Can you work these out from the model? Positions are in its coordinate system, mm. Face numbers are marked on the shaded views. A direction names the side the tool comes from. Give positions to 0.01 mm unless a question says otherwise; leave off trailing zeros. Order: outer loops, then holes, each group sorted by start corner. A loop starts at its lowest first (then second) coordinate and runs counter-clockwise, first axis right, second up. Notation, with made-up numbers: M -36,-8.75 L -16,-8.75 A8 ccw -16,-3.75 Z; hole C 33,75 d6. An arc over 180 degrees is marked long. One line per question, with ' | ' between items. Start each with the question number.
1) Thinking about a two-plate mould opening in Z: for the marked faces 4, 5 and 6, which applies, +Z half, -Z half, draft (parallel to the pull), parting line (faces both ways), or undercut?
2) If we section it at C-C, the plane x = 2.25: Please give me the cut outline in (y, z), plus the area to 3 significant figures.
3) If we section it at D-D, the plane y = 24: Please give me the cut outline in (x, z).
4) Please list where these lines run through material, in increasing order: line 1 along Y through (x, z) = (5.25, -4); line 2 along Y through (x, z) = (3, -7.5); line 3 along X through (y, z) = (9, -15). Write a range as [from, to].
5) I'm going to push flat-ended pins straight in: pin 1 Ø1.5 at (y, z) = (23, -5) entering from +X; pin 2 Ø1.5 at (y, z) = (7.5, -33) entering from +X; pin 3 Ø3 at (x, y) = (2, 10.5) entering from -Z; pin 4 Ø6 at (x, y) = (2, 10) entering from +Z. Where does each tip first touch, or does it pass through?
6) For the marked faces 1, 2 and 3, which set-ups out of +Z, -Z, +X, -X, +Y, -Y let a thin tool reach every point of the face, with its end or its side?
7) If we section it at B-B, the plane y = 11.25: State how many separate pieces and enclosed holes the cut face has, plus the area to 3 significant figures.
8) If we section it at A-A, the plane z = -8: Please give me the cut outline in (x, y), plus the area to 3 significant figures.
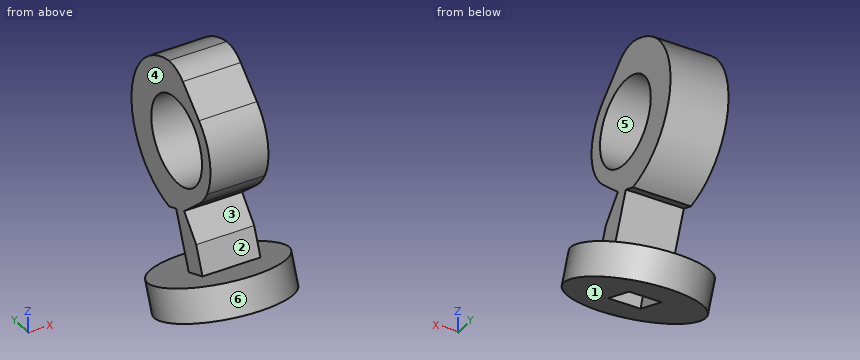
```python
from build123d import *

# Parameters (mm, degrees)
SKETCH1_R           = 6.750001985
BOSS_EXTRUDE1_DEPTH = 9
SKETCH3_R           = 10.000000826
BOSS_EXTRUDE2_DEPTH = 14
SKETCH4_R           = 10.000000826
SKETCH4_W           = 9
SKETCH4_H           = 8.939675258
CUT_EXTRUDE1_DEPTH  = 9
SKETCH5_W           = 9
SKETCH5_H           = 9
CUT_EXTRUDE2_DEPTH  = 3
SKETCH6_W           = 9
SKETCH6_H           = 9
CUT_EXTRUDE4_DEPTH  = 2
CUT_EXTRUDE5_DEPTH  = 10
SKETCH8_W           = 5
SKETCH8_H           = 6
CUT_EXTRUDE6_DEPTH  = 3


with BuildPart() as part:
    # Sketch1 → Boss-Extrude1 (new body)
    with BuildSketch(Plane(origin=(0, 0, 0), x_dir=(0, 0, -1), z_dir=(1, 0, 0))):
        with BuildLine():
            Line((-0.454941956, 12.359391949), (3.344728948, 8.050966095))
            ThreePointArc((3.344728948, 8.050966095), (8.344592491, 5.175709333), (14.063217322, 5.92608719))
            ThreePointArc((14.063217322, 5.92608719), (15.54600466, 6.868056536), (16.844733397, 8.050963212))
            Line((16.844733397, 8.050963212), (20.330899398, 12.003905107))
            Line((20.330899398, 12.003905107), (21.92689244, 16.003905107))
            ThreePointArc((21.92689244, 16.003905107), (10.143848092, 26.003055139), (-1.689188798, 16.063116838))
            ThreePointArc((-1.689188798, 16.063116838), (-1.448481266, 14.085815778), (-0.454941956, 12.359391949))
        make_face()
        with Locations((10.094731316, 14.003903077)):
            Circle(SKETCH1_R, mode=Mode.SUBTRACT)
    extrude(amount=BOSS_EXTRUDE1_DEPTH)

    # Sketch3 → Boss-Extrude2 (add)
    with BuildSketch(Plane(origin=(0, -5.349360366, -13.40697666), x_dir=(-1, 0, 0), z_dir=(0, -0.3705884577579875, -0.9287971764473427))):
        with Locations(Location((-4, 19.907031212, 0), (0, 0, 90))):
            Circle(SKETCH3_R)
    extrude(amount=BOSS_EXTRUDE2_DEPTH)

    # Sketch4 → Cut-Extrude1 (cut)
    with BuildSketch(Plane(origin=(0, -5.349360366, -13.40697666), x_dir=(1, 0, 0), z_dir=(0, 0.3705884577579875, 0.9287971764473427))):
        with Locations(Location((4, 19.907031212, 0), (0, 0, 270))):
            Circle(SKETCH4_R)
        with Locations((4.5, 19.495062719)):
            Rectangle(SKETCH4_W, SKETCH4_H, mode=Mode.SUBTRACT)
    extrude(amount=-CUT_EXTRUDE1_DEPTH, mode=Mode.SUBTRACT)

    # Sketch5 → Cut-Extrude2 (cut)
    with BuildSketch(Plane(origin=(0, 22.258531777, -8.88111546), x_dir=(1, 0, 0), z_dir=(0, 0.9287971764473427, -0.3705884577579875))):
        with Locations((4.5, 18.934773275)):
            Rectangle(SKETCH5_W, SKETCH5_H)
    extrude(amount=-CUT_EXTRUDE2_DEPTH, mode=Mode.SUBTRACT)

    # Sketch6 → Cut-Extrude4 (cut)
    with BuildSketch(Plane(origin=(0, 13.955386639, -5.568174994), x_dir=(1, 0, 0), z_dir=(0, -0.9287971764473427, 0.3705884577579875))):
        with Locations((4.5, -18.934773275)):
            Rectangle(SKETCH6_W, SKETCH6_H)
    extrude(amount=-CUT_EXTRUDE4_DEPTH, mode=Mode.SUBTRACT)

    # Sketch7 → Cut-Extrude5 (cut)
    with BuildSketch(Plane.ZY):
        Polygon((-20.330899398, 12.003905107), (-23.895915863, 8.795972566), (-19.716328569, 10.463620626), align=None)
    extrude(amount=-CUT_EXTRUDE5_DEPTH, mode=Mode.SUBTRACT)

    # Sketch8 → Cut-Extrude6 (cut)
    with BuildSketch(Plane(origin=(0, -10.537598775, -26.41013713), x_dir=(-1, 0, 0), z_dir=(0, -0.3705884577579875, -0.9287971764473427))):
        with Locations((-4, 19.907031212)):
            Rectangle(SKETCH8_W, SKETCH8_H)
    extrude(amount=-CUT_EXTRUDE6_DEPTH, mode=Mode.SUBTRACT)


solid = part.part
```
Results found:
1) face 4: draft | face 5: undercut | face 6: parting line
2) outline: M -1.19,-30.14 L 5.17,-32.68 L 6.28,-29.89 L 11.85,-32.11 L 10.74,-34.9 L 17.1,-37.44 L 18.95,-32.79 L 10.79,-29.54 L 14.12,-21.18 L 16,-21.93 A11.98 ccw 16.06,1.69 A5 ccw 12.36,0.45 L 8.05,-3.34 A9 ccw 5.93,-14.06 A10.18 ccw 8.05,-16.84 L 12,-20.33 L 8.8,-23.9 L 7.13,-28.08 L 0.66,-25.49 Z; hole C 14,-10.09 d13.5 | area: 332 mm²
3) outline: M 0,-16.74 L 9,-16.74 L 9,-3.48 L 0,-3.48 Z
4) line 1: y = [7.38, 11.1], [16.91, 24.33] | line 2: y = [5.39, 7.77], [20.24, 25.71] | line 3: x = [0, 9]
5) pin 1: stops at x = 9 | pin 2: stops at x = 14 | pin 3: stops at z = -35.4 | pin 4: stops at z = 0.93
6) face 1: -Z, +X, -X, -Y | face 2: +X, -X | face 3: +X, -X, -Y
7) separate pieces: 4 | enclosed holes: 1 | area: 221 mm²
8) outline: M 0,5.25 L 9,5.25 L 9,7.59 L 0,7.59 Z; M 0,20.42 L 9,20.42 L 9,25.82 L 0,25.82 Z | area: 69.6 mm²
